Can you work these out from the model? Positions are in its coordinate system, mm. Face numbers are marked on the shaded views. A direction names the side the tool comes from. Give positions to 0.01 mm unless a question says otherwise; leave off trailing zeros. Loops run counter-clockwise (first coordinate to the right, second up) from the corner with the lowest first, then second, coordinate; pieces in that order, holes last. Notation, with made-up numbers: (18.25, 29) -> (50.25, 29) arc R24 ccw to (50.25, 55) -> close; hole circle Ø11 at (-1, 12.25). An arc over 180 degrees is marked (long way). Return JSON: item names as keys, results as strings. Group by question number.
Q1. Which directions (+Z, -Z, +X, -X, +Y, -Y) give clear straight access to the entire face, cutting with the end or side of a thin tool? Please do the marked faces 1 and 2.
Q2. Suppose I cut it at B-B, the plane y = 7.5. Please give me the cut outline in (x, z), and give its area (3 significant figures).
Q3. I need wall thicknesses on line 1 along X through (y, z) = (35.85, 31.75); line 2 along Y through (x, z) = (11.75, 43.5); line 3 along Y through (x, z) = (1, 10). Which ranges of each line are inside material? Lowest first, please. Write a range as [from, to].
Q4. Suppose I cut it at D-D, the plane x = 14.75. Please give me the cut outline in (y, z).
Q5. Will these pins go through, and if not, where does the flat tip stop? pin 1 (9 mm diameter, centred on y = 24.21, z = 7.68, fed in from +X); pin 2 (3 mm diameter, centred on x = 5, z = 25, fed in from -Y).
Q6. Suppose I cut it at A-A, the plane z = 31.75. Please give me the cut outline in (x, y).
Q7. Suppose I cut it at C-C, the plane z = 39.75. Please give me the cut outline in (x, y).
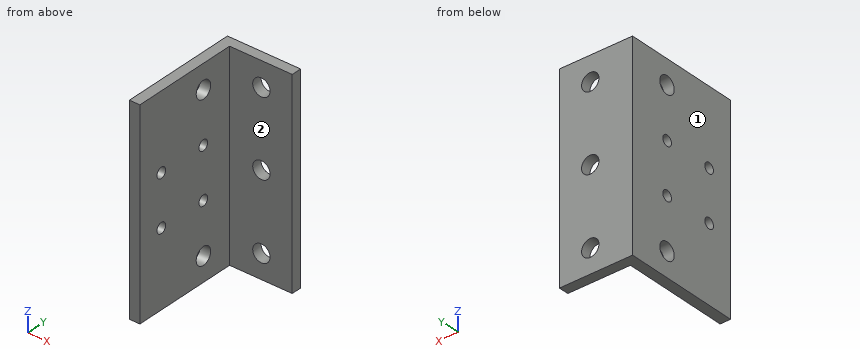
```python
from build123d import *

# Parameters (mm, degrees)
BOSS_EXTRUDE1_DEPTH         = 63.5
M5_CLEARANCE_HOLE1_D        = 5.5
M5_CLEARANCE_HOLE2_D        = 5.5
M5_CLEARANCE_HOLE3_D        = 5.5
M5_CLEARANCE_HOLE4_D        = 5.5
M5_CLEARANCE_HOLE5_D        = 5.5
TAP_DRILL_FOR_M4X0_7_TAP2_D = 3.3


with BuildPart() as part:
    # Sketch1 → Boss-Extrude1 (new body)
    with BuildSketch(Plane.XY):
        Polygon((0, 0), (0, 37.338), (23.114, 37.338), (23.114, 34.163), (3.302, 34.163), (3.302, 0), align=None)
    extrude(amount=BOSS_EXTRUDE1_DEPTH)

    # M5 Clearance Hole1 (through all)
    with Locations(Plane.ZY):
        with Locations((55.84134748, 24.208221519)):
            Hole(M5_CLEARANCE_HOLE1_D / 2)

    # M5 Clearance Hole2 (through all)
    with Locations(Plane.ZY):
        with Locations((7.677638483, 24.208221519)):
            Hole(M5_CLEARANCE_HOLE2_D / 2)

    # M5 Clearance Hole3 (through all)
    with Locations(Plane(origin=(0, 37.338, 0), x_dir=(1, 0, 0), z_dir=(0, 1, 0))):
        with Locations((13.368582087, -31.75)):
            Hole(M5_CLEARANCE_HOLE3_D / 2)

    # M5 Clearance Hole4 (through all)
    with Locations(Plane(origin=(0, 37.338, 0), x_dir=(1, 0, 0), z_dir=(0, 1, 0))):
        with Locations((13.368582087, -55.713693276)):
            Hole(M5_CLEARANCE_HOLE4_D / 2)

    # M5 Clearance Hole5 (through all)
    with Locations(Plane(origin=(0, 37.338, 0), x_dir=(1, 0, 0), z_dir=(0, 1, 0))):
        with Locations((13.368582087, -7.610649616)):
            Hole(M5_CLEARANCE_HOLE5_D / 2)

    # Tap Drill for M4x0.7 Tap2 (through all)
    with Locations(Plane.ZY):
        with Locations((23.75, 24.163), (23.75, 8.163), (39.75, 8.163), (39.75, 24.163)):
            Hole(TAP_DRILL_FOR_M4X0_7_TAP2_D / 2)


solid = part.part
```
Ans:
{
 "1": {"face 1": "+Z, -Z, -X, +Y, -Y", "face 2": "+Z, -Z, +X, -Y"},
 "2": {"outline": "(0, 0) -> (3.3, 0) -> (3.3, 22.24) -> (0, 22.24) -> close; (0, 25.26) -> (3.3, 25.26) -> (3.3, 38.24) -> (0, 38.24) -> close; (0, 41.26) -> (3.3, 41.26) -> (3.3, 63.5) -> (0, 63.5) -> close", "area": "190 mm^2"},
 "3": {"line 1": "x = [0, 10.62], [16.12, 23.11]", "line 2": "y = [34.16, 37.34]", "line 3": "y = [0, 22.74], [25.68, 37.34]"},
 "4": {"outline": "(34.16, 0) -> (37.34, 0) -> (37.34, 5.23) -> (34.16, 5.23) -> close; (34.16, 9.99) -> (37.34, 9.99) -> (37.34, 29.37) -> (34.16, 29.37) -> close; (34.16, 34.13) -> (37.34, 34.13) -> (37.34, 53.34) -> (34.16, 53.34) -> close; (34.16, 58.09) -> (37.34, 58.09) -> (37.34, 63.5) -> (34.16, 63.5) -> close"},
 "5": {"pin 1": "stops at x = 3.3", "pin 2": "stops at y = 34.16"},
 "6": {"outline": "(0, 0) -> (3.3, 0) -> (3.3, 34.16) -> (10.62, 34.16) -> (10.62, 37.34) -> (0, 37.34) -> close; (16.12, 34.16) -> (23.11, 34.16) -> (23.11, 37.34) -> (16.12, 37.34) -> close"},
 "7": {"outline": "(0, 0) -> (3.3, 0) -> (3.3, 6.51) -> (0, 6.51) -> close; (0, 9.81) -> (3.3, 9.81) -> (3.3, 22.51) -> (0, 22.51) -> close; (0, 25.81) -> (3.3, 25.81) -> (3.3, 34.16) -> (23.11, 34.16) -> (23.11, 37.34) -> (0, 37.34) -> close"}
}
